from build123d import *

# Parameters (mm, degrees)
PAD_DEPTH            = 40
SKETCH001_R          = 4
POCKET_DEPTH         = 50.001
POCKET_DEPTH_BACK    = -50.001
SKETCH002_R          = 2.25
POCKET001_DEPTH      = 37.001
POCKET001_DEPTH_BACK = -0.001
FILLET_R             = 3


with BuildPart() as part:
    # Sketch → Pad (new body, symmetric)
    with BuildSketch(Plane.XY):
        Polygon((-50, 0), (50, 0), (50, 37), (48, 37), (48, 2), (-48, 2), (-48, 37), (-50, 37), align=None)
    extrude(amount=PAD_DEPTH, both=True)

    # Sketch001 → Pocket (cut, two sides)
    with BuildSketch(Plane.YZ) as pocket_sk:
        with Locations((31, 25)):
            Circle(SKETCH001_R)
        with Locations((31, -25)):
            Circle(SKETCH001_R)
    extrude(amount=-POCKET_DEPTH, mode=Mode.SUBTRACT)
    extrude(pocket_sk.sketch, amount=-POCKET_DEPTH_BACK, mode=Mode.SUBTRACT)

    # Sketch002 → Pocket001 (cut, two sides)
    with BuildSketch(Plane.XZ) as pocket001_sk:
        with Locations((-4.5, 20)):
            Circle(SKETCH002_R)
        with Locations((4.5, 20)):
            Circle(SKETCH002_R)
        with Locations((-4.5, -20)):
            Circle(SKETCH002_R)
        with Locations((4.5, -20)):
            Circle(SKETCH002_R)
    extrude(amount=-POCKET001_DEPTH, mode=Mode.SUBTRACT)
    extrude(pocket001_sk.sketch, amount=-POCKET001_DEPTH_BACK, mode=Mode.SUBTRACT)

    # Fillet
    fillet_edges = [part.edges().sort_by_distance(p)[0] for p in [
        (48, 2, 0),
        (-48, 2, 0),
        (50, 0, 0),
        (-50, 0, 0),
    ]]
    fillet(fillet_edges, radius=FILLET_R)


solid = part.part
For this review, take the finished solid that the model builds, in its own axes (mm). A direction names the side the tool comes from. Round coordinates to 2 decimals unless told otherwise and drop trailing zeros. Loops run counter-clockwise (first coordinate to the right, second up) from the corner with the lowest first, then second, coordinate; pieces in that order, holes last. Notation, with made-up numbers: (86.5, -29) - (132.5, -29) arc R22 ccw to (132.5, -5) - close; hole circle Ø9 at (51, -8). An arc over 180 degrees is marked (long way). Put each result on its own line as item: value. Start each with the question number.
1. Consider section C-C on y = 31. State the section outline as (x, z) points.
2. Consider section A-A on x = 4.5. State the section outline as (y, z) points.
3. For probe 1 along Z at (x, y) = (48.4, 31); probe 2 along X at (y, z) = (13, -33.5); probe 3 along Z at (x, y) = (4.5, 1.45), list the stretches that pass through material, from the lowest coordinate up. Write a range as [from, to].
4. For faces 4 (the cylindrical face through (-47.1, 2.86, 0.56)), 5 (the cylindrical face through (-48.986, 30.479, 28.966)), list the 3-axis set-ups (+Z, -Z, +X, -X, +Y, -Y) from which the entire face can be reached by the end or side of a thin tool; tool diameter is ignored.
5. Mouldability with a two-part tool opening along X and no side actions: class faces 1 (the cylindrical face through (49.1, 0.86, 0.56)), 2 (the cylindrical face through (-48.99, 28.05, -22.3)), 3 (the flat face through (1, 2, 1)) as +X half, -X half, draft (parallel to the pull), parting line (faces both ways), or undercut.
6. Consider section D-D on y = 7.5. State the section outline as (x, z) points.
7. Consider section B-B on z = -25. State the section outline as (x, y) points.
8. Insertion check: P1, Ø2.5, axis at x = 4.5, z = 20, coming from the +Y side; P2, Ø6, axis at x = -4.5, z = 20, coming from the +Y side. Each pin has a flat end and moves straight along its axis. Give the tip position at first contact, or say it passes through.
Result sheet:
1. outline: (-50, -40) - (-48, -40) - (-48, -29) - (-50, -29) - close; (-50, -21) - (-48, -21) - (-48, 21) - (-50, 21) - close; (-50, 29) - (-48, 29) - (-48, 40) - (-50, 40) - close; (48, -40) - (50, -40) - (50, -29) - (48, -29) - close; (48, -21) - (50, -21) - (50, 21) - (48, 21) - close; (48, 29) - (50, 29) - (50, 40) - (48, 40) - close
2. outline: (0, -40) - (2, -40) - (2, -22.25) - (0, -22.25) - close; (0, -17.75) - (2, -17.75) - (2, 17.75) - (0, 17.75) - close; (0, 22.25) - (2, 22.25) - (2, 40) - (0, 40) - close
3. probe 1: [-40, -29], [-21, 21], [29, 40]
3. probe 2: [-50, -48], [48, 50]
3. probe 3: [-40, -22.25], [-17.75, 17.75], [22.25, 40]
4. face 4: +Z, -Z, +Y
4. face 5: +X, -X
5. face 1: +X half
5. face 2: draft
5. face 3: undercut
6. outline: (-50, -40) - (-48, -40) - (-48, 40) - (-50, 40) - close; (48, -40) - (50, -40) - (50, 40) - (48, 40) - close
7. outline: (-50, 3) arc R3 ccw to (-47, 0) - (47, 0) arc R3 ccw to (50, 3) - (50, 27) - (48, 27) - (48, 5) arc R3 cw to (45, 2) - (-45, 2) arc R3 cw to (-48, 5) - (-48, 27) - (-50, 27) - close; (-50, 35) - (-48, 35) - (-48, 37) - (-50, 37) - close; (48, 35) - (50, 35) - (50, 37) - (48, 37) - close
8. P1: through
8. P2: y = 2
